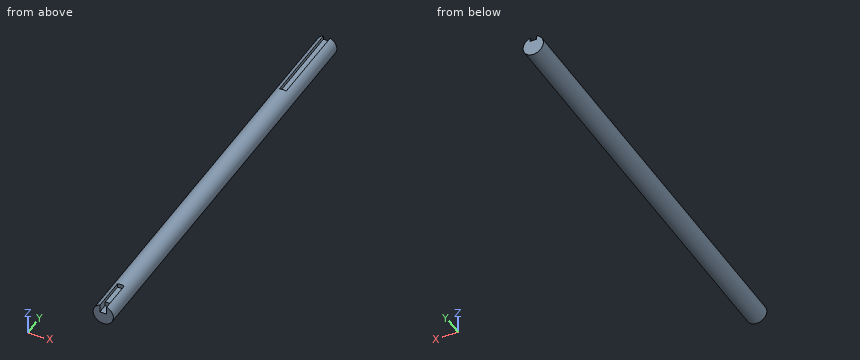
```python
from build123d import *

# Parameters (mm, degrees)
SKETCH1_R               = 6
BOSS_EXTRUDE1_DEPTH     = 254
SKETCH2_W               = 4
SKETCH2_H               = 5
CUT_EXTRUDE3_DEPTH      = 20
CUT_EXTRUDE3_DEPTH_BACK = 0.0001
CUT_EXTRUDE4_START      = 254
SKETCH2_2_W             = 4
SKETCH2_2_H             = 5
CUT_EXTRUDE4_DEPTH      = 50
SKETCH3_W               = 4
SKETCH3_H               = 10
CUT_EXTRUDE6_DEPTH      = 6


with BuildPart() as part:
    # Sketch1 → Boss-Extrude1 (new body)
    with BuildSketch(Plane(origin=(0, 0, 0), x_dir=(1, 0, 0), z_dir=(0, 1, 0))):
        Circle(SKETCH1_R)
    extrude(amount=BOSS_EXTRUDE1_DEPTH)

    # Sketch2 → Cut-Extrude3 (cut, two sides)
    with BuildSketch(Plane(origin=(0, 0, 0), x_dir=(1, 0, 0), z_dir=(0, 1, 0))) as cut_extrude3_sk:
        with Locations((0, -6)):
            Rectangle(SKETCH2_W, SKETCH2_H)
    extrude(amount=CUT_EXTRUDE3_DEPTH, mode=Mode.SUBTRACT)
    extrude(cut_extrude3_sk.sketch, amount=-CUT_EXTRUDE3_DEPTH_BACK, mode=Mode.SUBTRACT)

    # Sketch2<2> → Cut-Extrude4 (cut)
    with BuildSketch(Plane(origin=(0, 0, 0), x_dir=(1, 0, 0), z_dir=(0, 1, 0)).offset(CUT_EXTRUDE4_START)):
        with Locations((0, -6)):
            Rectangle(SKETCH2_2_W, SKETCH2_2_H)
    extrude(amount=-CUT_EXTRUDE4_DEPTH, mode=Mode.SUBTRACT)

    # Sketch3 → Cut-Extrude6 (cut)
    with BuildSketch(Plane(origin=(0, 0, 0), x_dir=(1, 0, 0), z_dir=(0, 1, 0))):
        with Locations((0, -6)):
            Rectangle(SKETCH3_W, SKETCH3_H)
    extrude(amount=CUT_EXTRUDE6_DEPTH, mode=Mode.SUBTRACT)


solid = part.part
```
Geometry: final body of the model. Coordinates: model frame, mm. Round coordinates to 2 decimals unless told otherwise and drop trailing zeros. Order: outer loops, then holes, each group sorted by start corner. A loop starts at its lowest first (then second) coordinate and runs counter-clockwise, first axis right, second up. Notation, with made-up numbers: (80, -3) - (112, -3) arc R23 ccw to (112, 34) - close; hole circle Ø1 at (-5, -3). An arc over 180 degrees is marked (long way). Use CSV: the item, a comma, the result in double quotes. Start each with the question number.
Q1. Section query B-B (y = 214.5). Return loops of the section in (x, z).
Q2. Section query D-D (y = 65.5). Return loops of the section in (x, z), and give its area (3 significant figures).
Q3. Material intervals for line 1 along Z through (x, y) = (-0.25, 115); line 2 along X through (y, z) = (169, -0.75); line 3 along Y through (x, z) = (-0.75, 4.5), sorted ascending. Write a range as from..to.
Q4. Section query C-C (z = -2). Return loops of the section in (x, y).
Q5. Section query A-A (x = 0). Return loops of the section in (y, z), and give its area (3 significant figures).
Q6. First-contact query: pin 1 (2 mm diameter, centred on x = 0, y = 220.5, fed in from +Z); pin 2 (2 mm diameter, centred on x = -3.5, y = 179, fed in from +Z); pin 3 (1.1 mm diameter, centred on y = 240, z = 4.5, fed in from -X). Flat tips, straight axial feed; report the tip coordinate or a pass-through.
Result set:
1,outline,"(-2, 3.5) - (-2, 5.66) arc R6 ccw (long way) to (2, 5.66) - (2, 3.5) - close"
2,outline,"circle Ø12 at (0, 0)"
2,area,"113 mm2"
3,line 1,"z = -5.99..5.99"
3,line 2,"x = -5.95..5.95"
3,line 3,"y = 20..204"
4,outline,"(-5.66, 0) - (5.66, 0) - (5.66, 254) - (-5.66, 254) - close"
5,outline,"(0, -6) - (254, -6) - (254, 3.5) - (204, 3.5) - (204, 6) - (20, 6) - (20, 3.5) - (6, 3.5) - (6, 1) - (0, 1) - close"
5,area,"2,860 mm2"
6,pin 1,"stops at z = 3.5"
6,pin 2,"stops at z = 5.45"
6,pin 3,"stops at x = -4.52"
